from build123d import *

# Parameters (mm, degrees)
BOSS_EXTRUDE1_DEPTH      = 15
BOSS_EXTRUDE1_DEPTH_BACK = 15
SKETCH2_R                = 10.375
CUT_EXTRUDE1_DEPTH       = 6.5


with BuildPart() as part:
    # Sketch1 → Boss-Extrude1 (new, two sides: drawn at the far end of the back side and taken through both)
    with BuildSketch(Plane.XY.offset(-BOSS_EXTRUDE1_DEPTH_BACK)):
        Polygon((-20, 6.5), (-20, 0), (-13.25, 0), (-14.5, -9), (-14.5, -24), (14.5, -24), (14.5, -9), (13.25, 0), (20, 0), (20, 6.5), align=None)
    extrude(amount=BOSS_EXTRUDE1_DEPTH + BOSS_EXTRUDE1_DEPTH_BACK)

    # Sketch2 → Cut-Extrude1 (cut)
    with BuildSketch(Plane(origin=(0, 6.5, 0), x_dir=(1, 0, 0), z_dir=(0, 1, 0))):
        with Locations(Location((0, 0, 0), (0, 0, 270))):
            Circle(SKETCH2_R)
    extrude(amount=-CUT_EXTRUDE1_DEPTH, mode=Mode.SUBTRACT)


solid = part.part
Could you check a few things on this model? Use its own coordinates, in mm. A direction names the side the tool comes from. Coordinates: 2 decimals unless noted, no trailing zeros. Order: outer loops, then holes, each group sorted by start corner. A loop starts at its lowest first (then second) coordinate and runs counter-clockwise, first axis right, second up. Notation, with made-up numbers: (26.25, -14.5) - (75.25, -14.5) arc R19 cw to (75.25, 19.5) - close; hole circle Ø8 at (-16, -31). An arc over 180 degrees is marked (long way). Answer in a Markdown table with one row per item. Add a question column.
(1) If we section it at D-D, the plane z = -6.5: Please give me the cut outline in (x, y).
(2) If we section it at B-B, the plane x = 9: Please give me the cut outline in (y, z), then the cut area to 3 significant figures.
(3) On a 3-axis mill with a long thin cutter (end or side, diameter ignored), from which of +Z, -Z, +X, -X, +Y, -Y can I reach the whole of each face in a straight line? I mean faces 4 (the face through (14.5, -17, 0)), 5 (the face through (17, 0, 0)), 6 (the face through (-13.866, -4.437, -0.21)), 7 (the face through (0, 0, 0)). Say none if no direction works.
(4) Will these pins go through, and if not, where does the flat tip stop? pin 1 (2 mm diameter, centred on y = -14.5, z = 5.5, fed in from -X); pin 2 (1.5 mm diameter, centred on x = -3, z = 0.5, fed in from +Y); pin 3 (7.5 mm diameter, centred on x = 16, z = 0, fed in from -Y); pin 4 (4.5 mm diameter, centred on y = -13.5, z = -6.5, fed in from +X).
(5) I need wall thicknesses on L1, parallel to X at y = 5.25, z = 0 (3 decimals); L2, parallel to X at y = -17.5, z = 9; L3, parallel to Y at x = -6, z = 3. Which ranges of each line are inside material? Lowest first, please.
(6) If we mould it in two halves opening along X, with no side actions, what happens to faces 1 (the face through (-17, 0, 0)), 2 (the face through (20, 3, 0)), 3 (the face through (3.1, 3.3, 9.9))? For each: released by +X, released by -X, zero draft, split by the parting line, or undercut.
(7) If we section it at C-C, the plane y = -11: Please give me the cut outline in (x, z).
(8) If we section it at A-A, the plane z = 0: Please give me the cut outline in (x, y) (3 decimals).
Results are:
| question | item | result |
|---|---|---|
| 1 | outline | (-20, 0) - (-13.25, 0) - (-14.5, -9) - (-14.5, -24) - (14.5, -24) - (14.5, -9) - (13.25, 0) - (20, 0) - (20, 6.5) - (8.09, 6.5) - (8.09, 0) - (-8.09, 0) - (-8.09, 6.5) - (-20, 6.5) - close |
| 2 | outline | (-24, -15) - (6.5, -15) - (6.5, -5.16) - (0, -5.16) - (0, 5.16) - (6.5, 5.16) - (6.5, 15) - (-24, 15) - close |
| 2 | area | 848 mm2 |
| 3 | face 4 | +Z, -Z, +X, -Y |
| 3 | face 5 | +Z, -Z, +X |
| 3 | face 6 | +Z, -Z, -X |
| 3 | face 7 | +Y |
| 4 | pin 1 | stops at x = -14.5 |
| 4 | pin 2 | stops at y = 0 |
| 4 | pin 3 | stops at y = -24 |
| 4 | pin 4 | stops at x = 14.5 |
| 5 | L1 | x = -20 to -10.375, 10.375 to 20 |
| 5 | L2 | x = -14.5 to 14.5 |
| 5 | L3 | y = -24 to 0 |
| 6 | face 1 | zero draft |
| 6 | face 2 | released by +X |
| 6 | face 3 | undercut |
| 7 | outline | (-14.5, -15) - (14.5, -15) - (14.5, 15) - (-14.5, 15) - close |
| 8 | outline | (-20, 0) - (-13.25, 0) - (-14.5, -9) - (-14.5, -24) - (14.5, -24) - (14.5, -9) - (13.25, 0) - (20, 0) - (20, 6.5) - (10.375, 6.5) - (10.375, 0) - (-10.375, 0) - (-10.375, 6.5) - (-20, 6.5) - close |
